Geometry check sheet. Reference: the model listing, model coordinates, mm. A direction names the side the tool comes from. Give positions to 0.01 mm unless a question says otherwise; leave off trailing zeros. Put each result on its own line as item: value. Start each with the question number.
Q1. Access from +Z, -Z, +X, -X, +Y, -Y to the whole of each face (thin tool, end or side, straight path). Record for faces 1 (the flat face through (460, 170, 25)), 2 (the flat face through (-460, -170, 25)), 3 (the flat face through (460, -170, 25)), 4 (the flat face through (-6, -200, 25)), 5 (the flat face through (-445, 185, 25)).
Q2. Go/stop test with flat-tipped pins: pin 1 (5 mm diameter, centred on y = -174, z = 5, fed in from -X); pin 2 (2.5 mm diameter, centred on y = 174, z = 5, fed in from +X); pin 3 (3 mm diameter, centred on y = -196, z = 45, fed in from -X). Record where each tip stops, or that it passes through.
Q3. Material ranges on L1, parallel to Z at x = -423, y = -174; L2, parallel to Y at x = 421, z = 45, recorded low to high.
Q4. Mould release check, pull along X, two halves, no side actions. Record for faces 6 (the flat face through (-475, -2, 25)), 7 (the flat face through (475, -2, 25)), 8 (the flat face through (-7, 3, 0)): +X half, -X half, draft (parallel to the pull), parting line (faces both ways), or undercut.
```python
from build123d import *

# Parameters (mm, degrees)
SKETCH1_W                 = 950
SKETCH1_H                 = 400
BOSS_EXTRUDE1_DEPTH       = 50
SKETCH2_W                 = 30
SKETCH2_H                 = 30
CUT_EXTRUDE1_DEPTH        = 518.80787943
F_4_0MM_DOWEL_HOLE1_D     = 4
F_4_0MM_DOWEL_HOLE1_DEPTH = 30
F_4_0MM_DOWEL_HOLE1_TIP   = 1.201721238
F_4_0MM_DOWEL_HOLE2_D     = 4
F_4_0MM_DOWEL_HOLE2_DEPTH = 30
F_4_0MM_DOWEL_HOLE2_TIP   = 1.201721238
F_4_0MM_DOWEL_HOLE3_D     = 4
F_4_0MM_DOWEL_HOLE3_DEPTH = 30
F_4_0MM_DOWEL_HOLE3_TIP   = 1.201721238
F_4_0MM_DOWEL_HOLE4_D     = 4
F_4_0MM_DOWEL_HOLE4_DEPTH = 30
F_4_0MM_DOWEL_HOLE4_TIP   = 1.201721238


with BuildPart() as part:
    # Sketch1 → Boss-Extrude1 (new body)
    with BuildSketch(Plane.XY):
        Rectangle(SKETCH1_W, SKETCH1_H)
    extrude(amount=BOSS_EXTRUDE1_DEPTH)

    # Sketch2 → Cut-Extrude1 (cut, through all)
    with BuildSketch(Plane.XY.offset(50)):
        with Locations((-460, 185)):
            Rectangle(SKETCH2_W, SKETCH2_H)
        with Locations((-460, -185)):
            Rectangle(SKETCH2_W, SKETCH2_H)
        with Locations((460, -185)):
            Rectangle(SKETCH2_W, SKETCH2_H)
        with Locations((460, 185)):
            Rectangle(SKETCH2_W, SKETCH2_H)
    extrude(amount=-CUT_EXTRUDE1_DEPTH, mode=Mode.SUBTRACT)

    # Ø4.0mm Dowel Hole1
    with Locations(Plane(origin=(445, -196, 45), x_dir=(0, 0, 1), z_dir=(1, 0, 0))):
        with Locations((0, 0), (0, -22), (-40, 0), (-40, -22)):
            Hole(F_4_0MM_DOWEL_HOLE1_D / 2, depth=F_4_0MM_DOWEL_HOLE1_DEPTH)
            with Locations((0, 0, -(F_4_0MM_DOWEL_HOLE1_DEPTH + F_4_0MM_DOWEL_HOLE1_TIP / 2))):  # 118° drill point
                Cone(0, F_4_0MM_DOWEL_HOLE1_D / 2, F_4_0MM_DOWEL_HOLE1_TIP, mode=Mode.SUBTRACT)

    # Ø4.0mm Dowel Hole2
    with Locations(Plane(origin=(-445, -174, 5), x_dir=(0, 0, -1), z_dir=(-1, 0, 0))):
        with Locations((0, 0), (-40, 0), (-40, 22), (0, 22)):
            Hole(F_4_0MM_DOWEL_HOLE2_D / 2, depth=F_4_0MM_DOWEL_HOLE2_DEPTH)
            with Locations((0, 0, -(F_4_0MM_DOWEL_HOLE2_DEPTH + F_4_0MM_DOWEL_HOLE2_TIP / 2))):  # 118° drill point
                Cone(0, F_4_0MM_DOWEL_HOLE2_D / 2, F_4_0MM_DOWEL_HOLE2_TIP, mode=Mode.SUBTRACT)

    # Ø4.0mm Dowel Hole3
    with Locations(Plane(origin=(-445, 174, 45), x_dir=(0, 0, -1), z_dir=(-1, 0, 0))):
        with Locations((0, 0), (0, -22), (40, -22), (40, 0)):
            Hole(F_4_0MM_DOWEL_HOLE3_D / 2, depth=F_4_0MM_DOWEL_HOLE3_DEPTH)
            with Locations((0, 0, -(F_4_0MM_DOWEL_HOLE3_DEPTH + F_4_0MM_DOWEL_HOLE3_TIP / 2))):  # 118° drill point
                Cone(0, F_4_0MM_DOWEL_HOLE3_D / 2, F_4_0MM_DOWEL_HOLE3_TIP, mode=Mode.SUBTRACT)

    # Ø4.0mm Dowel Hole4
    with Locations(Plane(origin=(445, 174, 45), x_dir=(0, 0, 1), z_dir=(1, 0, 0))):
        with Locations((0, 0), (0, -22), (-40, 0), (-40, -22)):
            Hole(F_4_0MM_DOWEL_HOLE4_D / 2, depth=F_4_0MM_DOWEL_HOLE4_DEPTH)
            with Locations((0, 0, -(F_4_0MM_DOWEL_HOLE4_DEPTH + F_4_0MM_DOWEL_HOLE4_TIP / 2))):  # 118° drill point
                Cone(0, F_4_0MM_DOWEL_HOLE4_D / 2, F_4_0MM_DOWEL_HOLE4_TIP, mode=Mode.SUBTRACT)


solid = part.part
```
Results found:
1. face 1: +Z, -Z, +X, +Y
1. face 2: +Z, -Z, -X, -Y
1. face 3: +Z, -Z, +X, -Y
1. face 4: +Z, -Z, +X, -X, -Y
1. face 5: +Z, -Z, -X, +Y
2. pin 1: stops at x = -445
2. pin 2: stops at x = 414.55
2. pin 3: stops at x = -414.7
3. L1: z = 0 to 3, 7 to 43, 47 to 50
3. L2: y = -200 to -198, -194 to -176, -172 to 172, 176 to 194, 198 to 200
4. face 6: -X half
4. face 7: +X half
4. face 8: draft
